```python
from build123d import *

# Parameters (mm, degrees)
F0_R     = 45.72
F1_DEPTH = 76.2
F3_DEPTH = 30.48


with BuildPart() as f1:
    # F0 (on Right) → F1 (new body)
    with BuildSketch(Plane.YZ):
        Circle(F0_R)
    extrude(amount=F1_DEPTH)

    # F2 (on face) → F3 (join)
    with BuildSketch(Plane.YZ.offset(76.2)):
        Polygon((-26.396454, -45.72), (26.396454, -45.72), (52.792909, 0), (26.396454, 45.72), (-26.396454, 45.72), (-52.792909, 0), align=None)
    extrude(amount=F3_DEPTH)

    # F4: F1 across plane


with BuildPart() as f1_1:
    add(f1.part)
    add(f1.part.mirror(Plane.YZ))


solid = f1_1.part
```
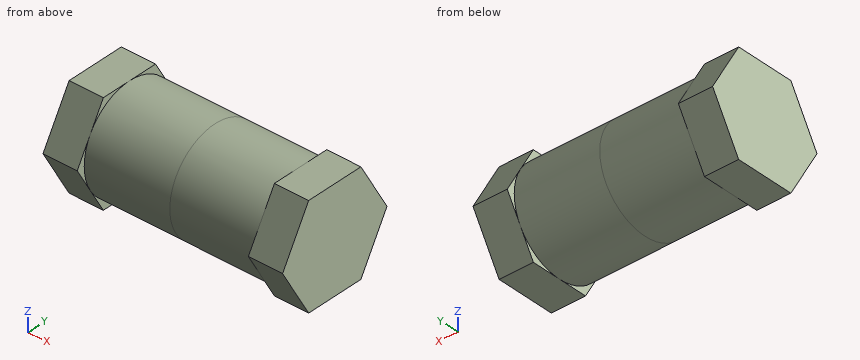
The model under review builds one solid part; all positions refer to its coordinate system, in mm. Round coordinates to 2 decimals unless told otherwise and drop trailing zeros. Loops run counter-clockwise (first coordinate to the right, second up) from the corner with the lowest first, then second, coordinate; pieces in that order, holes last.
1) Wall thickness on line 1 along Y through (x, z) = (21.5, -8.5); line 2 along Z through (x, y) = (51, 9.5); line 3 along Z through (x, y) = (3, 12): over which ranges is each line inside the solid? List them lowest first.
Values follow:
line 1: y = -44.92 to 44.92
line 2: z = -44.72 to 44.72
line 3: z = -44.12 to 44.12
2) Clearance check with flat-ended pins moving along their axes: P1, Ø10.5, axis at y = 47, z = -10.5, coming from the -X side; P2, Ø6, axis at x = 25.5, z = -30, coming from the -Y side; P3, Ø1.5, axis at x = 15.5, y = -15, coming from the +Z side; P4, Ø8, axis at x = -10.5, z = 28, coming from the +Y side. State where each tip first meets the part, or that it passes through.
Values follow:
P1: stops at x = -106.68
P2: stops at y = -36.9
P3: stops at z = 43.44
P4: stops at y = 38.91
3) Consider section C-C on x = -59. State the section outline as (y, z) points.
Values follow:
outline: circle Ø91.44 at (0, 0)
4) Consider section A-A on y = -35.5. State the section outline as (x, z) points, then the cut area to 3 significant figures.
Values follow:
outline: (-106.68, -29.95) - (-76.2, -29.95) - (-76.2, -28.81) - (76.2, -28.81) - (76.2, -29.95) - (106.68, -29.95) - (106.68, 29.95) - (76.2, 29.95) - (76.2, 28.81) - (-76.2, 28.81) - (-76.2, 29.95) - (-106.68, 29.95) - close
area: 12,400 mm2
5) Consider section B-B on z = 28.5. State the section outline as (x, y) points.
Values follow:
outline: (-106.68, -36.34) - (-76.2, -36.34) - (-76.2, -35.75) - (76.2, -35.75) - (76.2, -36.34) - (106.68, -36.34) - (106.68, 36.34) - (76.2, 36.34) - (76.2, 35.75) - (-76.2, 35.75) - (-76.2, 36.34) - (-106.68, 36.34) - close
